Geometry check sheet. Reference: the model listing, model coordinates, mm. Give positions to 0.01 mm unless a question says otherwise; leave off trailing zeros. Loops run counter-clockwise (first coordinate to the right, second up) from the corner with the lowest first, then second, coordinate; pieces in that order, holes last. Notation, with made-up numbers: (36, 12.25) -> (57, 12.25) arc R12 cw to (57, 28.25) -> close; hole circle Ø9 at (42, 26.25). An arc over 180 degrees is marked (long way). One line per item, written item: value. Start each with the question number.
(1) Sectioned sample at B-B, the plane x = 20.5. Record the cut outline in (y, z), then the cut area to 3 significant figures.
(2) Gauge pin test, flat end, axial feed: pin 1 Ø1.7 at (x, y) = (1, 18) entering from +Z. Record the tip position at first contact, or that the pin passes through.
(3) Sectioned sample at A-A, the plane z = 73.5. Record the cut outline in (x, y), then the cut area to 3 significant figures.
(4) Scan lines: line 1 along Y through (x, z) = (23.5, 364.5); line 2 along X through (y, z) = (44, 527.05). Record each from-to range of solid material in increasing order. Write a range as from..to.
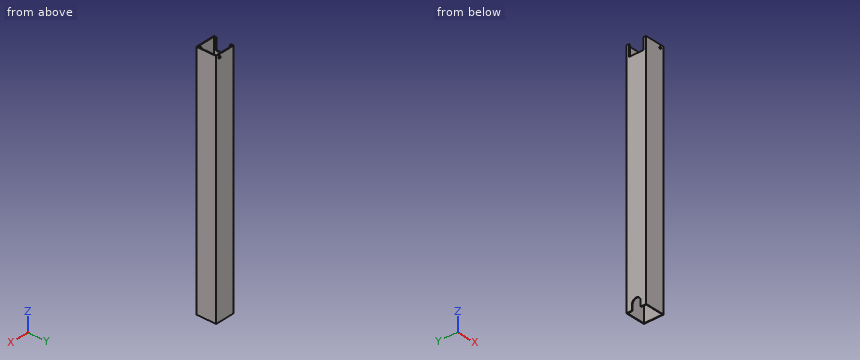
Autodesk Inventor part; units mm, degrees
ref_plane "YZ Plane" through (0, 0, 0) normal (1, 0, 0) x (0, 1, 0)
ref_plane "XZ Plane" through (0, 0, 0) normal (0, 1, 0) x (-1, 0, 0)
ref_plane "XY Plane" through (0, 0, 0) normal (0, 0, 1) x (1, 0, 0)
sketch "Sketch1" plane through (0, 0, 0) normal (0, 0, 1) x (1, 0, 0)
  line L0 (0, 0) -> (44.45, 0)
  line L1 (44.45, 0) -> (44.45, 44.45)
  line L2 (44.45, 44.45) -> (0, 44.45)
  line L3 (0, 44.45) -> (0, 0)
  line L4 (1.5875, 42.8625) -> (42.8625, 42.8625)
  line L5 (42.8625, 42.8625) -> (42.8625, 1.5875)
  line L6 (42.8625, 1.5875) -> (1.5875, 1.5875)
  line L7 (1.5875, 1.5875) -> (1.5875, 42.8625)
  dimension "d0" = 44.45
  dimension "d1" = 44.45
  dimension "d2" = 1.5875
extrude "Extrusion1" add sketch "Sketch1" along normal blind 533.4
sketch "Sketch2" plane through (44.45, 0, 0) normal (1, 0, 0) x (0, 0, -1)
  line L0 (0, 22.225) -> (-12.7, 22.225) construction
  line L1 (0, 12.7) -> (-12.7, 12.7)
  line L2 (-12.7, 31.75) -> (0, 31.75)
  arc A0 (0, 12.7) -> (0, 31.75) centre (0, 22.225) ccw
  arc A1 (-12.7, 31.75) -> (-12.7, 12.7) centre (-12.7, 22.225) ccw
  line L3 (0, 0) -> (0, 44.45)
  line L4 (0, 44.45) -> (-533.4, 44.45)
  point P0 (-6.35, 22.225)
  dimension "d5" = 0
  dimension "d7" = 19.05
  dimension "d20" = 12.7
  dimension "d21" = 22.225
extrude "Extrusion2" cut sketch "Sketch2" against normal blind 127
sketch "Sketch6" plane through (44.45, 0, 533.4) normal (1, 0, 0) x (0, 0, -1)
  line L0 (533.4, 42.8625) -> (533.4, 31.75)
  arc A0 (520.7, 31.75) -> (520.7, 12.7) centre (520.7, 22.225) ccw
  line L1 (533.4, 31.75) -> (520.7, 31.75)
  arc A1 (520.7, 31.75) -> (520.7, 12.7) centre (520.7, 22.225) ccw
  line L2 (533.4, 12.7) -> (520.7, 12.7)
  line L3 (520.7, 12.7) -> (533.4, 12.7)
  line L4 (533.4, 12.7) -> (533.4, 31.75)
  point P0 (533.4, 0)
extrude "Extrusion3" add sketch "Sketch6" against normal blind 1.5875
sketch "Sketch7" plane through (0, 0, 533.4) normal (-1, 0, 0) x (0, 0, 1)
  line L0 (0, 0) -> (0, 44.45)
  line L1 (0, 38.1) -> (-25.4, 38.1)
  line L2 (-25.4, 38.1) -> (-25.4, 6.35)
  line L3 (-25.4, 6.35) -> (0, 6.35)
  line L4 (0, 6.35) -> (0, 38.1)
  line L5 (-39.9502, 6.35) -> (-39.9502, 38.1)
  line L6 (-533.4, 31.75) -> (-520.7, 31.75)
  arc A0 (-520.7, 12.7) -> (-520.7, 31.75) centre (-520.7, 22.225) ccw
  line L7 (-520.7, 12.7) -> (-533.4, 12.7)
  line L8 (-533.4, 12.7) -> (-533.4, 0)
  line L9 (-533.4, 0) -> (0, 0)
  line L10 (0, 44.45) -> (0, 0)
  line L11 (-533.4, 44.45) -> (0, 44.45)
  line L12 (-533.4, 44.45) -> (-533.4, 31.75)
  dimension "d24" = 25.4
  dimension "d25" = 31.75
  dimension "d26" = 6.35
  dimension "d27" = 6.35
extrude "Extrusion4" cut sketch "Sketch7" against normal blind 1.5875 contours L3 L2 L1 L0
sketch "Sketch8" plane through (0, 0, 0) normal (0, -1, 0) x (1, 0, 0)
  line L0 (44.45, 0) -> (44.45, 533.4)
  line L1 (0, 533.4) -> (44.45, 533.4)
  point P0 (0, 0)
  point P1 (35.7188, 527.05)
  dimension "d30" = 8.7312
  dimension "d31" = 6.35
hole "Hole2" at (35.7188, 0, 527.05) direction (0, 1, 0) diameter 5.1562 depth 76.2 tip angle 118
equation "\"d26\" = d27"
properties part number "TelescopeOuter" material "Aluminum 6061"
Calculated:
1. outline: (0, 0) -> (1.59, 0) -> (1.59, 533.4) -> (0, 533.4) -> close; (42.86, 0) -> (44.45, 0) -> (44.45, 533.4) -> (42.86, 533.4) -> close
1. area: 1,690 mm2
2. pin 1: stops at z = 508
3. outline: (0, 0) -> (44.45, 0) -> (44.45, 44.45) -> (0, 44.45) -> close; hole (1.59, 1.59) -> (42.86, 1.59) -> (42.86, 42.86) -> (1.59, 42.86) -> close
3. area: 272 mm2
4. line 1: y = 0..1.59, 42.86..44.45
4. line 2: x = 0..33.14, 38.3..44.45
